Read the model definition and answer for the solid it produces. Units are mm, in the model's axes. Face numbers are marked on the shaded views. A direction names the side the tool comes from. Give positions to 0.01 mm unless a question says otherwise; leave off trailing zeros. Order: outer loops, then holes, each group sorted by start corner. A loop starts at its lowest first (then second) coordinate and runs counter-clockwise, first axis right, second up.
Item 1: The mould has two halves that part along X. Classify the marked faces 1, 2, 3 and 4: +X half, -X half, draft (parallel to the pull), parting line (faces both ways), or undercut.
Item 2: A cutting plane is placed at A-A (x = 0). Write down the section's boundary in (y, z).
Item 3: Find the intervals of material crossed by line 1 along Y through (x, z) = (0, 1.6); line 2 along Y through (x, z) = (2.45, 6.25); line 3 along Z through (x, y) = (-1.2, -1.75), in increasing order.
Item 4: Which of the six approach directions +Z, -Z, +X, -X, +Y, -Y give full straight-line access (tool end or side, diameter ignored) to the marked faces 5 and 6?
Item 5: A cutting plane is placed at D-D (z = 6.5). Write down the section's boundary in (x, y), plus the area to 3 significant figures.
Item 6: A cutting plane is placed at B-B (y = -0.75). Write down the section's boundary in (x, z).
Item 7: A cutting plane is placed at C-C (z = 2.5). Write down the section's boundary in (x, y), plus the area to 3 significant figures.
from build123d import *

# Parameters (mm, degrees)
F0_W     = 5.5
F0_H     = 5.5
F0_R     = 1.5
F0_H_2   = 2
F1_DEPTH = 3
F2_DEPTH = 8


with BuildPart() as f1:
    # F0 (on Top) → F1 (new body)
    with BuildSketch(Plane.XY):
        Rectangle(F0_W, F0_H)
        with Locations((0, -0.75)):
            Circle(F0_R, mode=Mode.SUBTRACT)
        with Locations((0, -3.75)):
            Rectangle(F0_W, F0_H_2)
    extrude(amount=F1_DEPTH)

    # F0 (on Top) → F2 (join)
    with BuildSketch(Plane.XY):
        with Locations((0, -3.75)):
            Rectangle(F0_W, F0_H_2)
    extrude(amount=F2_DEPTH)


solid = f1.part
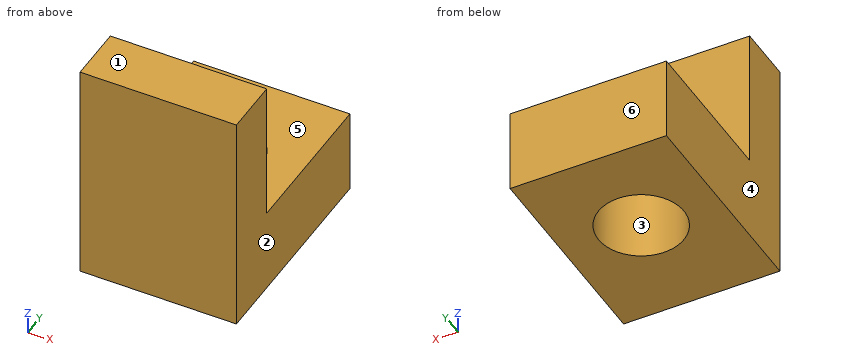
Response values:
1. face 1: draft
1. face 2: +X half
1. face 3: undercut
1. face 4: -X half
2. outline: (-4.75, 0) - (-2.25, 0) - (-2.25, 3) - (-2.75, 3) - (-2.75, 8) - (-4.75, 8) - close; (0.75, 0) - (2.75, 0) - (2.75, 3) - (0.75, 3) - close
3. line 1: y = -4.75 to -2.25, 0.75 to 2.75
3. line 2: y = -4.75 to -2.75
3. line 3: z = 0 to 3
4. face 5: +Z, +X, -X, +Y
4. face 6: +Z, -Z, +X, -X, +Y
5. outline: (-2.75, -4.75) - (2.75, -4.75) - (2.75, -2.75) - (-2.75, -2.75) - close
5. area: 11.0 mm2
6. outline: (-2.75, 0) - (-1.5, 0) - (-1.5, 3) - (-2.75, 3) - close; (1.5, 0) - (2.75, 0) - (2.75, 3) - (1.5, 3) - close
7. outline: (-2.75, -4.75) - (2.75, -4.75) - (2.75, 2.75) - (-2.75, 2.75) - close; hole circle Ø3 at (0, -0.75)
7. area: 34.2 mm2
